Read the model definition and answer for the solid it produces. Units are mm, in the model's axes. A direction names the side the tool comes from. Round coordinates to 2 decimals unless told otherwise and drop trailing zeros. Order: outer loops, then holes, each group sorted by start corner. A loop starts at its lowest first (then second) coordinate and runs counter-clockwise, first axis right, second up. Notation, with made-up numbers: (87, -19.75) -> (146, -19.75) arc R18 cw to (146, -15.75) -> close; hole circle Ø10 at (25, 79). An arc over 180 degrees is marked (long way). Answer as a JSON object with one key per item and string values. Group by question number.
Item 1: For faces 4 (the cylindrical face through (0.9, 0.74, -2.86)), 5 (the flat face through (6, 2, 22)), 6 (the flat face through (24, 0, 0)), 7 (the flat face through (0, 1, -23.619)), 8 (the flat face through (22, 1.2, 0)), determine the directions among +Z, -Z, +X, -X, +Y, -Y from which every point of the face is accessible in a straight line to the end or side of a thin tool.
Item 2: Section A-A, the plane x = -10 is taken. Write down the section's boundary in (y, z), plus the area to 3 significant figures.
Item 3: Section D-D, the plane x = -17 is taken. Write down the section's boundary in (y, z).
Item 4: Given P1, Ø1.5, axis at y = 1, z = 7, coming from the +X side; P2, Ø0.6, axis at x = -21.5, y = 1.5, coming from the +Z side; P3, Ø0.9, axis at x = 1, z = -23, coming from the -Y side; P4, Ø3, axis at x = -17.5, z = 13, coming from the +Y side, each flat-ended and moving along its own axis, determine where each tip first touches the part or whether it passes through.
Item 5: Section B-B, the plane z = 10 is taken. Write down the section's boundary in (x, y).
Item 6: Section C-C, the plane y = 2.2 is taken. Count the separate pieces of the cut face and the enclosed holes in it, plus the area to 3 significant figures.
Item 7: The mould has two halves that part along X. Classify faces 1 (the cylindrical face through (-5.3, 1.48, -24.17)), 2 (the cylindrical face through (6.36, 1.48, -19.35)), 3 (the flat face through (-20.619, 1, 0)): pulls with the +X half, pulls with the -X half, needs draft (parallel to the pull), parting line crosses it, or undercut.
Item 8: Consider probe 1 along X at (y, z) = (0.65, -3.5); probe 2 along X at (y, z) = (0.95, -5); probe 3 along Y at (x, z) = (23, 4). Determine where each line is inside the solid, lowest interval first. Write a range as from..to.
from build123d import *

# Parameters (mm, degrees)
SKIZZE1_R                       = 19
SKIZZE1_R_2                     = 1.6
AUFSATZ_LINEAR_AUSTRAGEN1_DEPTH = 3
SKIZZE6_R                       = 3
SCHNITT_LINEAR_AUSTRAGEN2_DEPTH = 1.5
SKIZZE7_W                       = 3
SKIZZE7_H                       = 12
SKIZZE7_W_2                     = 12
SKIZZE7_H_2                     = 3
SCHNITT_LINEAR_AUSTRAGEN3_DEPTH = 1.2


with BuildPart() as part:
    # Skizze1 → Aufsatz-Linear austragen1 (new body)
    with BuildSketch(Plane(origin=(0, 0, 0), x_dir=(1, 0, 0), z_dir=(0, 1, 0))):
        with BuildLine():
            ThreePointArc((6, -20.493901532), (6.348554352, -19.365749382), (7.272727273, -18.630819574))
            ThreePointArc((7.272727273, -18.630819574), (14.142135624, -14.142135624), (18.630819574, -7.272727273))
            ThreePointArc((18.630819574, -7.272727273), (19.365749382, -6.348554352), (20.493901532, -6))
            Line((20.493901532, -6), (22.649503306, -6))
            ThreePointArc((22.649503306, -6), (23.93487248, -5.532261755), (24.619025332, -4.347826087))
            ThreePointArc((24.619025332, -4.347826087), (25, 0), (24.619025332, 4.347826087))
            ThreePointArc((24.619025332, 4.347826087), (23.93487248, 5.532261755), (22.649503306, 6))
            Line((22.649503306, 6), (20.493901532, 6))
            ThreePointArc((20.493901532, 6), (19.365749382, 6.348554352), (18.630819574, 7.272727273))
            ThreePointArc((18.630819574, 7.272727273), (14.142135624, 14.142135624), (7.272727273, 18.630819574))
            ThreePointArc((7.272727273, 18.630819574), (6.348554352, 19.365749382), (6, 20.493901532))
            Line((6, 20.493901532), (6, 22.649503306))
            ThreePointArc((6, 22.649503306), (5.532261755, 23.93487248), (4.347826087, 24.619025332))
            ThreePointArc((4.347826087, 24.619025332), (0, 25), (-4.347826087, 24.619025332))
            ThreePointArc((-4.347826087, 24.619025332), (-5.532261755, 23.93487248), (-6, 22.649503306))
            Line((-6, 22.649503306), (-6, 20.493901532))
            ThreePointArc((-6, 20.493901532), (-6.348554352, 19.365749382), (-7.272727273, 18.630819574))
            ThreePointArc((-7.272727273, 18.630819574), (-14.142135624, 14.142135624), (-18.630819574, 7.272727273))
            ThreePointArc((-18.630819574, 7.272727273), (-19.365749382, 6.348554352), (-20.493901532, 6))
            Line((-20.493901532, 6), (-22.649503306, 6))
            ThreePointArc((-22.649503306, 6), (-23.93487248, 5.532261755), (-24.619025332, 4.347826087))
            ThreePointArc((-24.619025332, 4.347826087), (-25, 0), (-24.619025332, -4.347826087))
            ThreePointArc((-24.619025332, -4.347826087), (-23.93487248, -5.532261755), (-22.649503306, -6))
            Line((-22.649503306, -6), (-20.493901532, -6))
            ThreePointArc((-20.493901532, -6), (-19.365749382, -6.348554352), (-18.630819574, -7.272727273))
            ThreePointArc((-18.630819574, -7.272727273), (-14.142135624, -14.142135624), (-7.272727273, -18.630819574))
            ThreePointArc((-7.272727273, -18.630819574), (-6.348554352, -19.365749382), (-6, -20.493901532))
            Line((-6, -20.493901532), (-6, -22.649503306))
            ThreePointArc((-6, -22.649503306), (-5.532261755, -23.93487248), (-4.347826087, -24.619025332))
            ThreePointArc((-4.347826087, -24.619025332), (0, -25), (4.347826087, -24.619025332))
            ThreePointArc((4.347826087, -24.619025332), (5.532261755, -23.93487248), (6, -22.649503306))
            Line((6, -22.649503306), (6, -20.493901532))
        make_face()
        Circle(SKIZZE1_R, mode=Mode.SUBTRACT)
        Circle(SKIZZE1_R)
        with Locations(Location((0, -10, 0), (0, 0, 270))):
            Circle(SKIZZE1_R_2, mode=Mode.SUBTRACT)
        with Locations(Location((-10, 0, 0), (0, 0, 270))):
            Circle(SKIZZE1_R_2, mode=Mode.SUBTRACT)
        with Locations(Location((10, 0, 0), (0, 0, 270))):
            Circle(SKIZZE1_R_2, mode=Mode.SUBTRACT)
        with Locations(Location((0, 10, 0), (0, 0, 270))):
            Circle(SKIZZE1_R_2, mode=Mode.SUBTRACT)
        with Locations(Location((0, 0, 0), (0, 0, 270))):
            Circle(SKIZZE1_R_2, mode=Mode.SUBTRACT)
    extrude(amount=AUFSATZ_LINEAR_AUSTRAGEN1_DEPTH)

    # Skizze6 → Schnitt-Linear austragen2 (cut)
    with BuildSketch(Plane.XZ):
        with Locations(Location((0, 0, 0), (0, 0, 270))):
            Circle(SKIZZE6_R)
    extrude(amount=-SCHNITT_LINEAR_AUSTRAGEN2_DEPTH, mode=Mode.SUBTRACT)

    # Skizze7 → Schnitt-Linear austragen3 (cut)
    with BuildSketch(Plane.XZ):
        with Locations((-22.119025332, 0)):
            Rectangle(SKIZZE7_W, SKIZZE7_H)
        with Locations((0, 22.119025332)):
            Rectangle(SKIZZE7_W_2, SKIZZE7_H_2)
        with Locations((22.119025332, 0)):
            Rectangle(SKIZZE7_W, SKIZZE7_H)
        with Locations((0, -22.119025332)):
            Rectangle(SKIZZE7_W_2, SKIZZE7_H_2)
    extrude(amount=-SCHNITT_LINEAR_AUSTRAGEN3_DEPTH, mode=Mode.SUBTRACT)


solid = part.part
Values found:
{
 "1": {"face 4": "-Y", "face 5": "+Z, +X, +Y, -Y", "face 6": "+Z, -Z, +X, -X, -Y", "face 7": "+X, -X, -Y", "face 8": "+Z, -Z, -Y"},
 "2": {"outline": "(0, -17.32) -> (3, -17.32) -> (3, -1.6) -> (0, -1.6) -> close; (0, 1.6) -> (3, 1.6) -> (3, 17.32) -> (0, 17.32) -> close", "area": "94.3 mm2"},
 "3": {"outline": "(0, -10.54) -> (3, -10.54) -> (3, 10.54) -> (0, 10.54) -> close"},
 "4": {"P1": "x = 19.53", "P2": "z = 6", "P3": "y = 1.2", "P4": "through"},
 "5": {"outline": "(-17.32, 0) -> (-1.6, 0) -> (-1.6, 3) -> (-17.32, 3) -> close; (1.6, 0) -> (17.32, 0) -> (17.32, 3) -> (1.6, 3) -> close"},
 "6": {"separate pieces": "1", "enclosed holes": "5", "area": "1,460 mm2"},
 "7": {"face 1": "pulls with the -X half", "face 2": "pulls with the +X half", "face 3": "undercut"},
 "8": {"probe 1": "-24.75..-23.62, -20.62..20.62, 23.62..24.75", "probe 2": "-24.38..-23.62, -20.62..20.62, 23.62..24.38", "probe 3": "1.2..3"}
}
